The listing builds one solid part. Answer for the finished solid, in the listing's coordinates (mm). Face numbers are marked on the shaded views. Coordinates: 2 decimals unless noted, no trailing zeros. Loops run counter-clockwise (first coordinate to the right, second up) from the corner with the lowest first, then second, coordinate; pieces in that order, holes last. Notation, with made-up numbers: M 80,1 L 95,1 A10 cw 95,5 Z; hole C 30.25,-9.5 d8. An arc over 180 degrees is marked long. Answer in a Markdown table with one row per item. Add a question column.
from build123d import *

# Parameters (mm, degrees)
BOSS_EXTRUDE1_DEPTH = 278
CUT_EXTRUDE3_REACH  = 287.279
SKETCH2_R           = 2


with BuildPart() as part:
    # Sketch1 → Boss-Extrude1 (new body)
    with BuildSketch(Plane(origin=(0, 0, 0), x_dir=(0, 0, -1), z_dir=(1, 0, 0))):
        Polygon((0, 0), (50, 0), (50, 45), (45, 45), (45, 5), (5, 5), (5, 45), (0, 45), align=None)
    extrude(amount=BOSS_EXTRUDE1_DEPTH)

    # Sketch2 → Cut-Extrude3 (cut, up to next)
    with BuildSketch(Plane(origin=(0, 5, 0), x_dir=(1, 0, 0), z_dir=(0, 1, 0)), mode=Mode.PRIVATE) as cut_extrude3_sk1:
        with Locations(Location((8, 15.475, 0), (0, 0, 270))):
            Circle(SKETCH2_R)
    cut_extrude3_tool1 = extrude(cut_extrude3_sk1.sketch, amount=-CUT_EXTRUDE3_REACH, mode=Mode.PRIVATE) & part.part
    # Sketch2 → Cut-Extrude3 (cut, up to next)
    with BuildSketch(Plane(origin=(0, 5, 0), x_dir=(1, 0, 0), z_dir=(0, 1, 0)), mode=Mode.PRIVATE) as cut_extrude3_sk2:
        with Locations(Location((55, 15.475, 0), (0, 0, 270))):
            Circle(SKETCH2_R)
    cut_extrude3_tool2 = extrude(cut_extrude3_sk2.sketch, amount=-CUT_EXTRUDE3_REACH, mode=Mode.PRIVATE) & part.part
    # Sketch2 → Cut-Extrude3 (cut, up to next)
    with BuildSketch(Plane(origin=(0, 5, 0), x_dir=(1, 0, 0), z_dir=(0, 1, 0)), mode=Mode.PRIVATE) as cut_extrude3_sk3:
        with Locations(Location((55, 34.525, 0), (0, 0, 270))):
            Circle(SKETCH2_R)
    cut_extrude3_tool3 = extrude(cut_extrude3_sk3.sketch, amount=-CUT_EXTRUDE3_REACH, mode=Mode.PRIVATE) & part.part
    # Sketch2 → Cut-Extrude3 (cut, up to next)
    with BuildSketch(Plane(origin=(0, 5, 0), x_dir=(1, 0, 0), z_dir=(0, 1, 0)), mode=Mode.PRIVATE) as cut_extrude3_sk4:
        with Locations(Location((8, 34.525, 0), (0, 0, 270))):
            Circle(SKETCH2_R)
    cut_extrude3_tool4 = extrude(cut_extrude3_sk4.sketch, amount=-CUT_EXTRUDE3_REACH, mode=Mode.PRIVATE) & part.part
    # Sketch2 → Cut-Extrude3 (cut, up to next)
    with BuildSketch(Plane(origin=(0, 5, 0), x_dir=(1, 0, 0), z_dir=(0, 1, 0)), mode=Mode.PRIVATE) as cut_extrude3_sk5:
        with Locations(Location((270, 34.525, 0), (0, 0, 270))):
            Circle(SKETCH2_R)
    cut_extrude3_tool5 = extrude(cut_extrude3_sk5.sketch, amount=-CUT_EXTRUDE3_REACH, mode=Mode.PRIVATE) & part.part
    # Sketch2 → Cut-Extrude3 (cut, up to next)
    with BuildSketch(Plane(origin=(0, 5, 0), x_dir=(1, 0, 0), z_dir=(0, 1, 0)), mode=Mode.PRIVATE) as cut_extrude3_sk6:
        with Locations(Location((223, 34.525, 0), (0, 0, 270))):
            Circle(SKETCH2_R)
    cut_extrude3_tool6 = extrude(cut_extrude3_sk6.sketch, amount=-CUT_EXTRUDE3_REACH, mode=Mode.PRIVATE) & part.part
    # Sketch2 → Cut-Extrude3 (cut, up to next)
    with BuildSketch(Plane(origin=(0, 5, 0), x_dir=(1, 0, 0), z_dir=(0, 1, 0)), mode=Mode.PRIVATE) as cut_extrude3_sk7:
        with Locations(Location((223, 15.475, 0), (0, 0, 270))):
            Circle(SKETCH2_R)
    cut_extrude3_tool7 = extrude(cut_extrude3_sk7.sketch, amount=-CUT_EXTRUDE3_REACH, mode=Mode.PRIVATE) & part.part
    # Sketch2 → Cut-Extrude3 (cut, up to next)
    with BuildSketch(Plane(origin=(0, 5, 0), x_dir=(1, 0, 0), z_dir=(0, 1, 0)), mode=Mode.PRIVATE) as cut_extrude3_sk8:
        with Locations(Location((270, 15.475, 0), (0, 0, 270))):
            Circle(SKETCH2_R)
    cut_extrude3_tool8 = extrude(cut_extrude3_sk8.sketch, amount=-CUT_EXTRUDE3_REACH, mode=Mode.PRIVATE) & part.part
    add(cut_extrude3_tool1.solids().sort_by_distance((8, 5, -15.475))[0], mode=Mode.SUBTRACT)
    add(cut_extrude3_tool2.solids().sort_by_distance((55, 5, -15.475))[0], mode=Mode.SUBTRACT)
    add(cut_extrude3_tool3.solids().sort_by_distance((55, 5, -34.525))[0], mode=Mode.SUBTRACT)
    add(cut_extrude3_tool4.solids().sort_by_distance((8, 5, -34.525))[0], mode=Mode.SUBTRACT)
    add(cut_extrude3_tool5.solids().sort_by_distance((270, 5, -34.525))[0], mode=Mode.SUBTRACT)
    add(cut_extrude3_tool6.solids().sort_by_distance((223, 5, -34.525))[0], mode=Mode.SUBTRACT)
    add(cut_extrude3_tool7.solids().sort_by_distance((223, 5, -15.475))[0], mode=Mode.SUBTRACT)
    add(cut_extrude3_tool8.solids().sort_by_distance((270, 5, -15.475))[0], mode=Mode.SUBTRACT)


solid = part.part
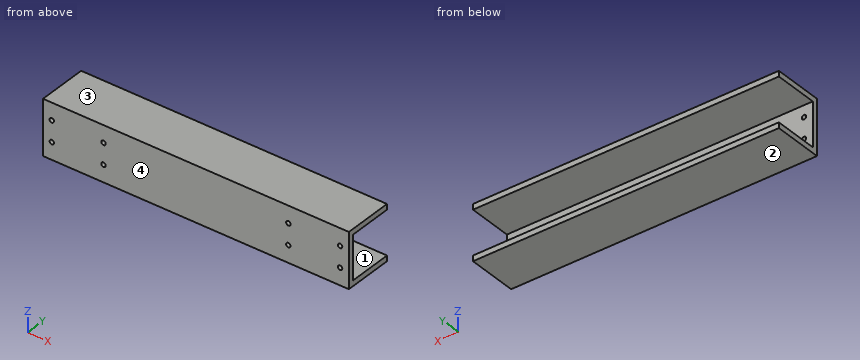
(1) Each of these flat-tipped pins is pushed along its axis until it touches: pin 1 (12 mm diameter, centred on y = 39.5, z = -11.5, fed in from +X); pin 2 (4.5 mm diameter, centred on x = 223, z = -34.525, fed in from +Y). Where does it stop, or does it pass through?
(2) A cutting plane is placed at B-B (x = 167). Give the vertices of the cut face in (y, z).
(3) The mould has two halves that part along Z. Classify the marked faces 1, 2, 3 and 4: released by +Z, released by -Z, zero draft, split by the parting line, or undercut.
(4) A cutting plane is placed at C-C (z = -25.5). Give the vertices of the cut face in (x, y).
(5) A cutting plane is placed at A-A (y = 30). Give the vertices of the cut face in (x, z), plus the area to 3 significant figures.
(6) Straight lines are drawn through the part: line 1 (Z direction, x = 270, y = 1) (3 decimals); line 2 (Z direction, x = 60.5, y = 21.5); line 3 (Y direction, x = 98, z = -17). For each, find the intervals that lie inside material, in ascending order.
Solved:
| question | item | result |
|---|---|---|
| 1 | pin 1 | passes through |
| 1 | pin 2 | stops at y = 5 |
| 2 | outline | M 0,-50 L 45,-50 L 45,-45 L 5,-45 L 5,-5 L 45,-5 L 45,0 L 0,0 Z |
| 3 | face 1 | undercut |
| 3 | face 2 | released by -Z |
| 3 | face 3 | released by +Z |
| 3 | face 4 | zero draft |
| 4 | outline | M 0,0 L 278,0 L 278,5 L 0,5 Z |
| 5 | outline | M 0,-50 L 278,-50 L 278,-45 L 0,-45 Z; M 0,-5 L 278,-5 L 278,0 L 0,0 Z |
| 5 | area | 2,780 mm² |
| 6 | line 1 | z = -50 to -36.525, -32.525 to -17.475, -13.475 to 0 |
| 6 | line 2 | z = -50 to -45, -5 to 0 |
| 6 | line 3 | y = 0 to 5 |
